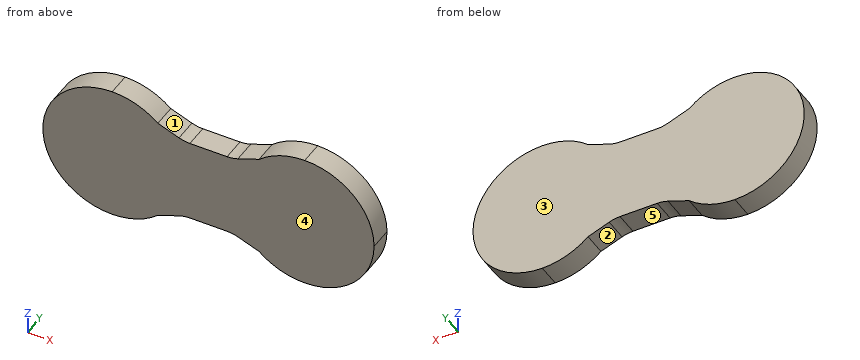
from build123d import *

# Parameters (mm, degrees)
F1_DEPTH = 19.05


with BuildPart() as f1:
    # F0 (on Front) → F1 (new body)
    with BuildSketch(Plane.XZ):
        with BuildLine():
            Line((20.027097595, 36.4074036121), (2.6105293283, 42.9636023111))
            ThreePointArc((2.6105293283, 42.9636023111), (16.9814393634, 23.5834144733), (22.0743066938, 0))
            ThreePointArc((22.0743066938, 0), (16.9814393634, -23.5834144733), (2.6105293283, -42.9636023111))
            Line((2.6105293283, -42.9636023111), (20.027097595, -36.4074036121))
            ThreePointArc((20.027097595, -36.4074036121), (24.4278254251, -35.189367606), (28.975523916, -34.7789341976))
            Line((28.975523916, -34.7789341976), (59.6230894717, -34.7789341976))
            ThreePointArc((59.6230894717, -34.7789341976), (64.1707879626, -35.189367606), (68.5715157927, -36.4074036121))
            Line((68.5715157927, -36.4074036121), (85.9880840594, -42.9636023111))
            ThreePointArc((85.9880840594, -42.9636023111), (66.5243066938, 0), (85.9880840594, 42.9636023111))
            Line((85.9880840594, 42.9636023111), (68.5715157927, 36.4074036121))
            ThreePointArc((68.5715157927, 36.4074036121), (64.1707879626, 35.189367606), (59.6230894717, 34.7789341976))
            Line((59.6230894717, 34.7789341976), (28.975523916, 34.7789341976))
            ThreePointArc((28.975523916, 34.7789341976), (24.4278254251, 35.189367606), (20.027097595, 36.4074036121))
        make_face()
        with BuildLine():
            ThreePointArc((2.6105293283, 42.9636023111), (-14.941734084, 53.4859438174), (-35.0756933062, 57.15))
            Line((-35.0756933062, 57.15), (2.6105293283, 42.9636023111))
        make_face()
        with BuildLine():
            Line((123.6743066938, 57.15), (85.9880840594, 42.9636023111))
            ThreePointArc((85.9880840594, 42.9636023111), (66.5243066938, 0), (85.9880840594, -42.9636023111))
            Line((85.9880840594, -42.9636023111), (123.6743066938, -57.15))
            ThreePointArc((123.6743066938, -57.15), (164.0854592386, -40.4111525448), (180.8243066938, 0))
            ThreePointArc((180.8243066938, 0), (164.0854592386, 40.4111525448), (123.6743066938, 57.15))
        make_face()
        with BuildLine():
            ThreePointArc((123.6743066938, 57.15), (103.5403474717, 53.4859438174), (85.9880840594, 42.9636023111))
            Line((85.9880840594, 42.9636023111), (123.6743066938, 57.15))
        make_face()
        with BuildLine():
            Line((2.6105293283, 42.9636023111), (-35.0756933062, 57.15))
            ThreePointArc((-35.0756933062, 57.15), (-92.2256933062, 0), (-35.0756933062, -57.15))
            Line((-35.0756933062, -57.15), (2.6105293283, -42.9636023111))
            ThreePointArc((2.6105293283, -42.9636023111), (16.9814393634, -23.5834144733), (22.0743066938, 0))
            ThreePointArc((22.0743066938, 0), (16.9814393634, 23.5834144733), (2.6105293283, 42.9636023111))
        make_face()
        with BuildLine():
            Line((2.6105293283, -42.9636023111), (-35.0756933062, -57.15))
            ThreePointArc((-35.0756933062, -57.15), (-14.941734084, -53.4859438174), (2.6105293283, -42.9636023111))
        make_face()
        with BuildLine():
            Line((123.6743066938, -57.15), (85.9880840594, -42.9636023111))
            ThreePointArc((85.9880840594, -42.9636023111), (103.5403474717, -53.4859438174), (123.6743066938, -57.15))
        make_face()
    extrude(amount=F1_DEPTH)


solid = f1.part
The listing builds one solid part. Answer for the finished solid, in the listing's coordinates (mm). Face numbers are marked on the shaded views. A direction names the side the tool comes from. Coordinates: 2 decimals unless noted, no trailing zeros. Write each loop counter-clockwise with the first axis right and the second up, starting at its lowest first coordinate (ties: lowest second). Pieces come first, ordered by that corner, then holes. Notation, with made-up numbers: M 50.25,8.5 L 76.25,8.5 A4 cw 76.25,12.5 Z; hole C -13,23.5 d10. An arc over 180 degrees is marked long. Put each result on its own line as item: value. Start each with the question number.
1. A cutting plane is placed at D-D on x = -57. Write down the section's boundary in (y, z), then the cut area to 3 significant figures.
2. A cutting plane is placed at A-A on z = -46.5. Write down the section's boundary in (x, y).
3. A cutting plane is placed at B-B on y = -11.75. Write down the section's boundary in (x, z).
4. Flat-ended cylindrical pins translate along their axes: P1, Ø3, axis at x = 108.5, z = -21, coming from the +Y side; P2, Ø10, axis at y = -11, z = 37, coming from the +X side; P3, Ø5, axis at x = 147.5, y = -10, coming from the +Z side; P4, Ø3, axis at y = -3.5, z = -26.5, coming from the +X side. Find the tip coordinate at first contact, or state that the pin passes through.
5. A cutting plane is placed at C-C on z = -32. Write down the section's boundary in (x, y).
6. For a pull along X with two mould halves and no side action, classify the marked faces 4 and 5 as pulls with the +X half, pulls with the -X half, needs draft (parallel to the pull), parting line crosses it, or undercut.
7. Which of the six approach directions +Z, -Z, +X, -X, +Y, -Y give full straight-line access (tool end or side, diameter ignored) to the marked faces 1, 2 and 3?
8. Consider line 1 (Z direction, x = 60, y = -15); line 2 (X direction, y = -9.75, z = 29); line 3 (Z direction, x = -81, y = -11.25). Determine where each line is inside the solid, lowest interval first. Write a range as from..to.
Resolved:
1. outline: M -19.05,-52.78 L 0,-52.78 L 0,52.78 L -19.05,52.78 Z
1. area: 2,010 mm2
2. outline: M -68.3,-19.05 L -1.85,-19.05 L -1.85,0 L -68.3,0 Z; M 90.45,-19.05 L 156.9,-19.05 L 156.9,0 L 90.45,0 Z
3. outline: M 2.61,-42.96 L 20.03,-36.41 A25.4 cw 28.98,-34.78 L 59.62,-34.78 A25.4 cw 68.57,-36.41 L 85.99,-42.96 A57.15 ccw long 85.99,42.96 L 68.57,36.41 A25.4 cw 59.62,34.78 L 28.98,34.78 A25.4 cw 20.03,36.41 L 2.61,42.96 A57.15 ccw long Z
4. P1: stops at y = 0
4. P2: stops at x = 171.03
4. P3: stops at z = 53.02
4. P4: stops at x = 175.07
5. outline: M -82.43,-19.05 L 171.03,-19.05 L 171.03,0 L -82.43,0 Z
6. face 4: needs draft
6. face 5: undercut
7. face 1: +Z, +Y, -Y
7. face 2: -Z, +Y, -Y
7. face 3: +Z, -Z, +X, -X, +Y
8. line 1: z = -34.78..34.78
8. line 2: x = -84.32..172.92
8. line 3: z = -34.02..34.02
